```python
from build123d import *

# Parameters (mm, degrees)
EXTRUDE_1_DEPTH     = 72
SKETCH_2_W          = 68.186813186
SKETCH_2_H          = 36
CUT_EXTRUDE_1_DEPTH = 10
SKETCH_3_W          = 5
SKETCH_3_H          = 36
CUT_EXTRUDE_3_DEPTH = 40
SKETCH_4_W          = 5
SKETCH_4_H          = 36
CUT_EXTRUDE_4_DEPTH = 40
EXTRUDE_2_DEPTH     = 5
EXTRUDE_3_DEPTH     = 67
SKETCH_8_W          = 52
SKETCH_8_H          = 38.074034261
CUT_EXTRUDE_5_DEPTH = 5


with BuildPart() as part:
    # 草圖1 → 填料-伸長1 (new body)
    with BuildSketch(Plane.XY):
        Polygon((-56.41038016, 13.571428571), (-56.41038016, -36.428571429), (-51.41038016, -36.428571429), (-51.41038016, -6.428571429), (16.776433026, -6.428571429), (16.776433026, -36.428571429), (21.776433026, -36.428571429), (21.776433026, 13.571428571), align=None)
    extrude(amount=EXTRUDE_1_DEPTH)

    # 草圖2 → 除料-伸長1 (cut)
    with BuildSketch(Plane.XZ.offset(6.428571429)):
        with Locations((-17.316973567, 32.5)):
            Rectangle(SKETCH_2_W, SKETCH_2_H)
    extrude(amount=-CUT_EXTRUDE_1_DEPTH, mode=Mode.SUBTRACT)

    # 草圖3 → 除料-伸長3 (cut)
    with BuildSketch(Plane.XZ.offset(36.428571429)):
        with Locations((-53.91038016, 32.5)):
            Rectangle(SKETCH_3_W, SKETCH_3_H)
    extrude(amount=-CUT_EXTRUDE_3_DEPTH, mode=Mode.SUBTRACT)

    # 草圖4 → 除料-伸長4 (cut)
    with BuildSketch(Plane.XZ.offset(36.428571429)):
        with Locations((19.276433026, 32.5)):
            Rectangle(SKETCH_4_W, SKETCH_4_H)
    extrude(amount=-CUT_EXTRUDE_4_DEPTH, mode=Mode.SUBTRACT)

    # 草圖5 → 填料-伸長2 (add)
    with BuildSketch(Plane.XY.offset(72)):
        Polygon((-56.41038016, 13.571428571), (-43.469427905, 61.867719886), (-38.469427905, 61.867719886), (-44.939904033, 37.719574229), (-26.587313333, 32.802012372), (-18.799180477, 61.867719886), (-11.799180477, 61.867719886), (-17.316973567, 37.484242705), (-17.316973567, 13.571428571), align=None)
    extrude(amount=-EXTRUDE_2_DEPTH)

    # 草圖7 → 填料-伸長3 (add)
    with BuildSketch(Plane(origin=(0, 0, 67), x_dir=(-1, 0, 0), z_dir=(0, 0, -1))):
        Polygon((17.316973567, 13.571428571), (31.740132733, 13.571428571), (26.587313333, 32.802012372), (18.799180477, 61.867719886), (11.799180477, 61.867719886), (17.316973567, 37.484242705), align=None)
        Polygon((31.740132733, 13.571428571), (56.41038016, 13.571428571), (43.469427905, 61.867719886), (38.469427905, 61.867719886), (44.939904033, 37.719574229), (50.092723432, 18.488990428), align=None)
    extrude(amount=EXTRUDE_3_DEPTH)

    # 草圖8 → 除料-伸長5 (cut)
    with BuildSketch(Plane(origin=(-56.024458351, 15.011708372, 0), x_dir=(0, 0, 1), z_dir=(-0.965925826, 0.258819045, 0))):
        with Locations((26, 32.545929761)):
            Rectangle(SKETCH_8_W, SKETCH_8_H)
    extrude(amount=-CUT_EXTRUDE_5_DEPTH, mode=Mode.SUBTRACT)


solid = part.part
```
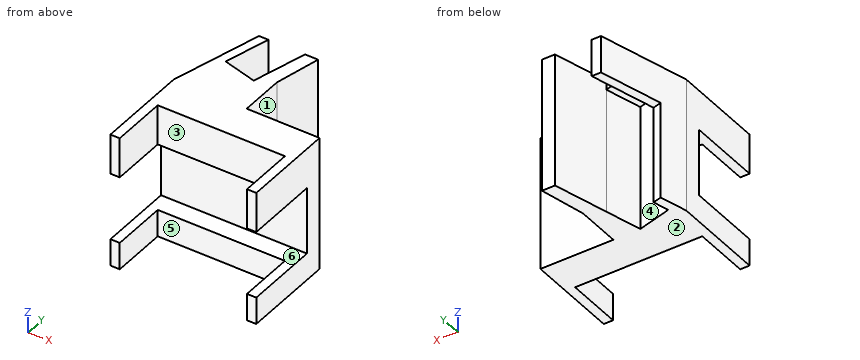
The listing builds one solid part. Answer for the finished solid, in the listing's coordinates (mm). Face numbers are marked on the shaded views. A direction names the side the tool comes from. Round coordinates to 2 decimals unless told otherwise and drop trailing zeros. Order: outer loops, then holes, each group sorted by start corner. A loop starts at its lowest first (then second) coordinate and runs counter-clockwise, first axis right, second up. Notation, with made-up numbers: (1.5, 58.5) - (50.5, 58.5) arc R26 cw to (50.5, 88.5) - close; hole circle Ø10 at (54.25, 38). An arc over 180 degrees is marked (long way). Put each result on its own line as item: value. Start each with the question number.
(1) Find section D-D (z = 53.5). Give the vertices of the cut face in (x, y).
(2) Find section A-A (y = -17). Give the vertices of the cut face in (x, z).
(3) Determine the mould class of the marked faces 1, 2 and 3 for opening direction Y: released by +Y, released by -Y, zero draft, split by the parting line, or undercut.
(4) Find section B-B (x = -14). Give the vertices of the cut face in (y, z).
(5) Given P1, Ø20, axis at x = -20.5, y = -15, coming from the +Z side; P2, Ø19, axis at x = -38, y = 28.5, coming from the -Z side; P3, Ø2, axis at x = -33.5, z = 49.5, coming from the +Y side; P4, Ø17, axis at x = -19.5, z = 66, coming from the -Y side, each flat-ended and moving along its own axis, determine where each tip first touches the part or whether it passes through.
(6) For the marked faces 4, 5 and 6, determine the directions among +Z, -Z, +X, -X, +Y, -Y from which every point of the face is accessible in a straight line to the end or side of a thin tool.
(7) Straight lines are drawn through the part: probe 1 along Z at (x, y) = (-49, -4); probe 2 along Y at (x, z) = (16, 3.5); probe 3 along Y at (x, z) = (18, 56). For each, find the intervals that lie inside material, in ascending order. Write a range as from..to.
(8) Find section C-C (y = 46). Give the vertices of the cut face in (x, z), plus the area to 3 significant figures.
Reply:
1. outline: (-56.41, -36.43) - (-51.41, -36.43) - (-51.41, -6.43) - (16.78, -6.43) - (16.78, -36.43) - (21.78, -36.43) - (21.78, 13.57) - (-17.32, 13.57) - (-17.32, 37.48) - (-11.8, 61.87) - (-18.8, 61.87) - (-31.74, 13.57) - (-50.09, 18.49) - (-38.47, 61.87) - (-43.47, 61.87) - (-56.41, 13.57) - close
2. outline: (-56.41, 0) - (-51.41, 0) - (-51.41, 14.5) - (-56.41, 14.5) - close; (-56.41, 50.5) - (-51.41, 50.5) - (-51.41, 72) - (-56.41, 72) - close; (16.78, 0) - (21.78, 0) - (21.78, 14.5) - (16.78, 14.5) - close; (16.78, 50.5) - (21.78, 50.5) - (21.78, 72) - (16.78, 72) - close
3. face 1: undercut
3. face 2: zero draft
3. face 3: released by -Y
4. outline: (-6.43, 0) - (13.57, 0) - (13.57, 72) - (-6.43, 72) - (-6.43, 50.5) - (3.57, 50.5) - (3.57, 14.5) - (-6.43, 14.5) - close; (52.14, 0) - (61.87, 0) - (61.87, 72) - (52.14, 72) - close
5. P1: z = 72
5. P2: z = 52
5. P3: y = 14.31
5. P4: y = -6.43
6. face 4: -Z
6. face 5: +Z, -Z, -Y
6. face 6: +X, -X, -Y
7. probe 1: 0..14.5, 50.5..72
7. probe 2: -6.43..13.57
7. probe 3: -36.43..13.57
8. outline: (-47.72, 52) - (-42.72, 52) - (-42.72, 72) - (-47.72, 72) - close; (-23.05, 0) - (-15.39, 0) - (-15.39, 72) - (-23.05, 72) - close
8. area: 652 mm^2
